Check sheet for the modelled part. Datum: model origin and axes. Units: mm. Face numbers are marked on the shaded views. A direction names the side the tool comes from. Coordinates: 2 decimals unless noted, no trailing zeros. Write each loop counter-clockwise with the first axis right and the second up, starting at its lowest first coordinate (ties: lowest second). Pieces come first, ordered by that corner, then holes. Notation, with made-up numbers: (75, 63.5) -> (85, 63.5) arc R21 ccw to (85, 67.5) -> close; hole circle Ø7 at (-14.5, -36). An arc over 180 degrees is marked (long way). Put each result on its own line as item: value.
```python
from build123d import *

# Parameters (mm, degrees)
BOSS_EXTRUDE1_DEPTH = 3
SKETCH2_R           = 1.5
CUT_EXTRUDE1_DEPTH  = 3
SKETCH3_W           = 24
SKETCH3_H           = 5
CUT_EXTRUDE2_DEPTH  = 1
SKETCH4_W           = 3
SKETCH4_H           = 30
BOSS_EXTRUDE2_DEPTH = 10
SKETCH5_R           = 1.5
CUT_EXTRUDE3_DEPTH  = 3


with BuildPart() as part:
    # Sketch1 → Boss-Extrude1 (new body)
    with BuildSketch(Plane(origin=(0, 0, 0), x_dir=(1, 0, 0), z_dir=(0, 1, 0))):
        Polygon((20, -11.899861304), (15, -11.899861304), (15, 18.100138696), (-15, 18.100138696), (-15, -11.899861304), (-20, -11.899861304), (-20, 23.100138696), (20, 23.100138696), align=None)
    extrude(amount=BOSS_EXTRUDE1_DEPTH)

    # Sketch2 → Cut-Extrude1 (cut)
    with BuildSketch(Plane(origin=(0, 3, 0), x_dir=(1, 0, 0), z_dir=(0, 1, 0))):
        with Locations(Location((-17.5, 3.100138696, 0), (0, 0, 90))):
            Circle(SKETCH2_R)
    extrude(amount=-CUT_EXTRUDE1_DEPTH, mode=Mode.SUBTRACT)

    # Sketch3 → Cut-Extrude2 (cut)
    with BuildSketch(Plane(origin=(0, 3, 0), x_dir=(1, 0, 0), z_dir=(0, 1, 0))):
        with Locations((0, 20.600138696)):
            Rectangle(SKETCH3_W, SKETCH3_H)
    extrude(amount=-CUT_EXTRUDE2_DEPTH, mode=Mode.SUBTRACT)

    # Sketch4 → Boss-Extrude2 (add)
    with BuildSketch(Plane(origin=(0, 3, 0), x_dir=(1, 0, 0), z_dir=(0, 1, 0))):
        with Locations((18.5, 3.100138696)):
            Rectangle(SKETCH4_W, SKETCH4_H)
    extrude(amount=BOSS_EXTRUDE2_DEPTH)

    # Sketch5 → Cut-Extrude3 (cut)
    with BuildSketch(Plane(origin=(0, 3, 0), x_dir=(1, 0, 0), z_dir=(0, 1, 0))):
        with Locations(Location((16, 20.600138696, 0), (0, 0, 270))):
            Circle(SKETCH5_R)
    extrude(amount=-CUT_EXTRUDE3_DEPTH, mode=Mode.SUBTRACT)


solid = part.part
```
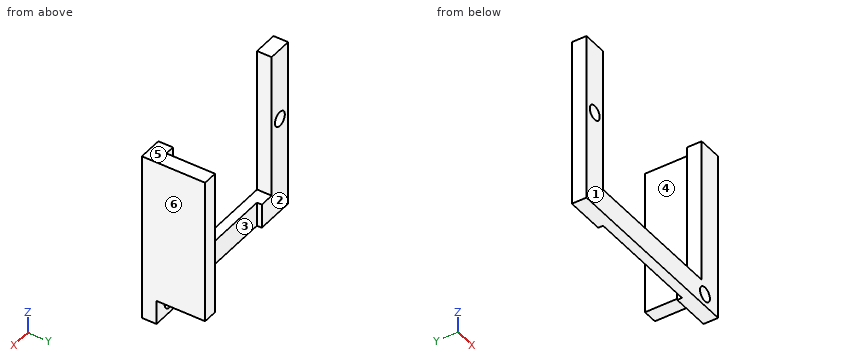
Q1. Material ranges on line 1 along Z through (x, y) = (-17.5, 1.15); line 2 along X through (y, z) = (1.25, -10.5); line 3 along X through (y, z) = (4, -8), recorded low to high.
Recorded:
line 1: z = -23.1 to -4.6, -1.6 to 11.9
line 2: x = -20 to -15, 15 to 20
line 3: x = 17 to 20
Q2. Depth check by flat-ended pin: P1, Ø5, axis at x = -17.5, z = -3.1, coming from the +Y side; P2, Ø1.5, axis at x = 0, y = 1.5, coming from the +Z side; P3, Ø1.5, axis at y = 8.5, z = -12, coming from the -X side; P4, Ø2.5, axis at x = 16.5, z = -10.5, coming from the +Y side. Enter the tip coordinate at first touch or a pass-through.
Recorded:
P1: stops at y = 3
P2: stops at z = -18.1
P3: stops at x = 17
P4: stops at y = 13
Q3. Mould release check, pull along X, two halves, no side actions. Record for the marked faces 3, 4, 5 and 6: released by +X, released by -X, zero draft, split by the parting line, or undercut.
Recorded:
face 3: undercut
face 4: released by -X
face 5: zero draft
face 6: released by +X
Q4. Cross-section at C-C (y = 1.5). Record the cut outline in (x, z).
Recorded:
outline: (-20, -23.1) -> (20, -23.1) -> (20, 11.9) -> (15, 11.9) -> (15, -18.1) -> (-15, -18.1) -> (-15, 11.9) -> (-20, 11.9) -> close; hole circle Ø3 at (-17.5, -3.1); hole circle Ø3 at (16, -20.6)
Q5. Cross-section at D-D (y = 3.5). Record the cut outline in (x, z).
Recorded:
outline: (17, -18.1) -> (20, -18.1) -> (20, 11.9) -> (17, 11.9) -> close
Q6. Tool access check on the marked faces 1 and 2. Record the directions out of +Z, -Z, +X, -X, +Y, -Y that give a thin tool (end or side, any length) a straight path to the whole face; none if there is none.
Recorded:
face 1: +Z, -Z, +X, -X, -Y
face 2: +Z, -Z, -X, +Y
Q7. Cross-section at A-A (x = 16). Record the cut outline in (y, z).
Recorded:
outline: (0, -23.1) -> (3, -23.1) -> (3, -22.1) -> (0, -22.1) -> close; (0, -19.1) -> (3, -19.1) -> (3, 11.9) -> (0, 11.9) -> close
Q8. Cross-section at B-B (z = 2). Record the cut outline in (x, y).
Recorded:
outline: (-20, 0) -> (-15, 0) -> (-15, 3) -> (-20, 3) -> close; (15, 0) -> (20, 0) -> (20, 13) -> (17, 13) -> (17, 3) -> (15, 3) -> close
